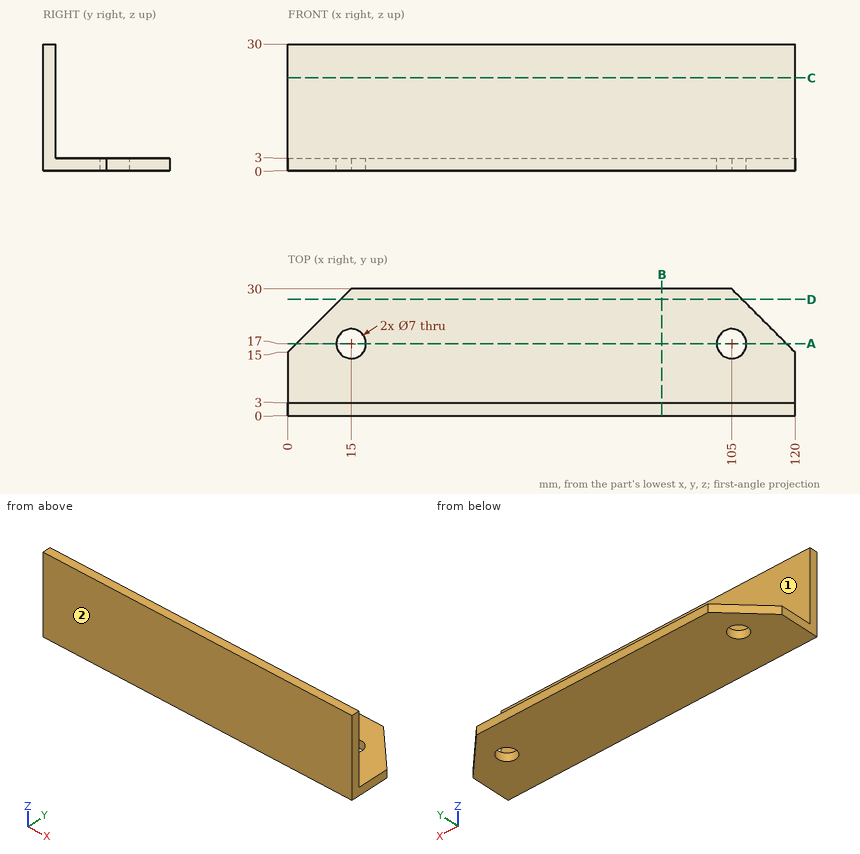
Source: three-view drawing plus pictorial views. Frame: mm from the lowest corner of the part. A direction names the side the tool comes from. Coordinates: 2 decimals unless noted, no trailing zeros. Loops run counter-clockwise (first coordinate to the right, second up) from the corner with the lowest first, then second, coordinate; pieces in that order, holes last. Notation, with made-up numbers: (-19, 74.25) - (-13, 74.25) arc R17 ccw to (-13, 87.25) - close; hole circle Ø4 at (41.25, 44). An arc over 180 degrees is marked (long way). One line per question, with ' | ' between items.
1) Section A-A, the plane y = 17. Return loops of the section in (x, z).
Report:
outline: (2, 0) - (11.5, 0) - (11.5, 3) - (2, 3) - close; (18.5, 0) - (101.5, 0) - (101.5, 3) - (18.5, 3) - close; (108.5, 0) - (118, 0) - (118, 3) - (108.5, 3) - close
2) First-contact query: P1, Ø8, axis at x = 33, y = 14.5, coming from the +Z side; P2, Ø8, axis at x = 84, z = 21, coming from the +Y side. Flat tips, straight axial feed; report the tip coordinate or a pass-through.
Report:
P1: stops at z = 3 | P2: stops at y = 3
3) Section B-B, the plane x = 88.5. Return loops of the section in (y, z), then the cut area to 3 significant figures.
Report:
outline: (0, 0) - (30, 0) - (30, 3) - (3, 3) - (3, 30) - (0, 30) - close | area: 171 mm²
4) Section D-D, the plane y = 27.5. Return loops of the section in (x, z), then the cut area to 3 significant figures.
Report:
outline: (12.5, 0) - (107.5, 0) - (107.5, 3) - (12.5, 3) - close | area: 285 mm²
5) Set-up query: the marked faces 1 and 2. Return all of +Z, -Z, +X, -X, +Y, -Y with unobstructed straight access to the full face (end or side cutting, diameter ignored); none if empty.
Report:
face 1: +Z, +X, -X, +Y | face 2: +Z, -Z, +X, -X, -Y
6) Line query: line 1 along Y through (x, z) = (15, 2.25); line 2 along Z through (x, y) = (70, 24). Output: solid intervals per line, ascending.
Report:
line 1: y = 0 to 13.5, 20.5 to 30 | line 2: z = 0 to 3
7) Section C-C, the plane z = 22. Return loops of the section in (x, y), then the cut area to 3 significant figures.
Report:
outline: (0, 0) - (120, 0) - (120, 3) - (0, 3) - close | area: 360 mm²
